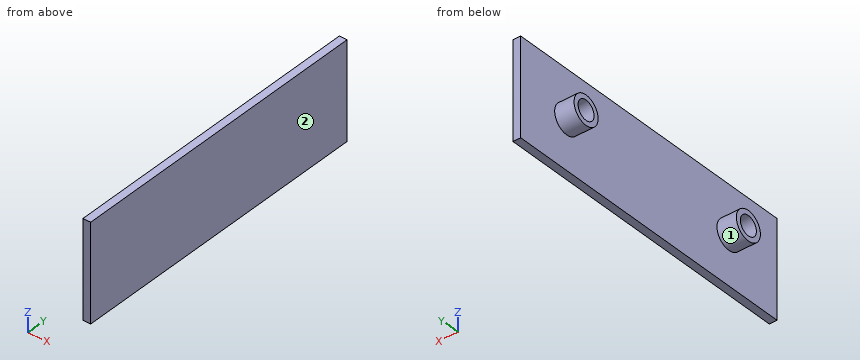
from build123d import *

# Parameters (mm, degrees)
SKETCH1_W           = 2.54
SKETCH1_H           = 31.75
BOSS_EXTRUDE1_DEPTH = 101.6
SKETCH5_R           = 4.7625
SKETCH5_R_2         = 3.175
BOSS_EXTRUDE3_DEPTH = 6.35


with BuildPart() as part:
    # Sketch1 → Boss-Extrude1 (new body)
    with BuildSketch(Plane(origin=(0, 0, 0), x_dir=(1, 0, 0), z_dir=(0, 1, 0))):
        with Locations((1.27, 15.875)):
            Rectangle(SKETCH1_W, SKETCH1_H)
    extrude(amount=BOSS_EXTRUDE1_DEPTH)

    # Sketch5 → Boss-Extrude3 (add)
    with BuildSketch(Plane(origin=(0, 0, 0), x_dir=(0, 0, -1), z_dir=(1, 0, 0))):
        with Locations((15.875, 19.05)):
            Circle(SKETCH5_R)
        with Locations((15.875, 19.05)):
            Circle(SKETCH5_R_2, mode=Mode.SUBTRACT)
        with Locations((15.875, 83.383819167)):
            Circle(SKETCH5_R)
        with Locations((15.875, 83.383819167)):
            Circle(SKETCH5_R_2, mode=Mode.SUBTRACT)
    extrude(amount=-BOSS_EXTRUDE3_DEPTH)


solid = part.part
Verification items for the finished model (mm, model axes). Face numbers are marked on the shaded views. A direction names the side the tool comes from. Coordinates: 2 decimals unless noted, no trailing zeros. Order: outer loops, then holes, each group sorted by start corner. A loop starts at its lowest first (then second) coordinate and runs counter-clockwise, first axis right, second up. Notation, with made-up numbers: (16, 28.25) -> (75, 28.25) arc R26 cw to (75, 54.25) -> close; hole circle Ø10 at (-22, 34). An arc over 180 degrees is marked (long way). Use CSV: the item, a comma, the result in double quotes. Start each with the question number.
Q1. Section check A-A, the plane x = -2.75. Give the number of separate pieces and of enclosed holes in the cut face, and give its area (3 significant figures).
Q2. Section check C-C, the plane z = -7.5. Record the cut outline in (x, y).
Q3. Section check D-D, the plane y = 71.5. Record the cut outline in (x, z).
Q4. Depth check by flat-ended pin: P1, Ø5, axis at y = 83.38, z = -15.88, coming from the -X side. Enter the tip coordinate at first touch or a pass-through.
Q5. Thickness scan on line 1 along X through (y, z) = (39.5, -18); line 2 along Y through (x, z) = (-1, -17.5); line 3 along Y through (x, z) = (-5.25, -20). Record the ranges inside material, lowest first.
Q6. Section check B-B, the plane y = 19.05. Record the cut outline in (x, z), and give its area (3 significant figures).
Q7. Tool access check on the marked faces 1 and 2. Record the directions out of +Z, -Z, +X, -X, +Y, -Y that give a thin tool (end or side, any length) a straight path to the whole face; none if there is none.
Returned:
1,separate pieces,"2"
1,enclosed holes,"2"
1,area,"79.2 mm^2"
2,outline,"(0, 0) -> (2.54, 0) -> (2.54, 101.6) -> (0, 101.6) -> close"
3,outline,"(0, -31.75) -> (2.54, -31.75) -> (2.54, 0) -> (0, 0) -> close"
4,P1,"stops at x = 0"
5,line 1,"x = 0 to 2.54"
5,line 2,"y = 14.57 to 16.32, 21.78 to 23.53, 78.91 to 80.66, 86.11 to 87.86"
5,line 3,"y = 16.67 to 21.43, 81 to 85.76"
6,outline,"(-6.35, -20.64) -> (0, -20.64) -> (0, -31.75) -> (2.54, -31.75) -> (2.54, 0) -> (0, 0) -> (0, -11.11) -> (-6.35, -11.11) -> (-6.35, -12.7) -> (0, -12.7) -> (0, -19.05) -> (-6.35, -19.05) -> close"
6,area,"101 mm^2"
7,face 1,"-X"
7,face 2,"+Z, -Z, +X, +Y, -Y"
